Verification items for the finished model (mm, model axes). Face numbers are marked on the shaded views. Give positions to 0.01 mm unless a question says otherwise; leave off trailing zeros. Loops run counter-clockwise (first coordinate to the right, second up) from the corner with the lowest first, then second, coordinate; pieces in that order, holes last. Notation, with made-up numbers: M 14,14 L 63,14 A16 cw 63,43 Z; hole C 46.25,12.25 d8. An arc over 180 degrees is marked long. Put each result on its own line as item: value. Start each with the question number.
from build123d import *

# Parameters (mm, degrees)
F1_DEPTH = 10
F0_R     = 24.5
F2_DEPTH = 150
F4_D     = 8.5
F4_DEPTH = 31.001
F5_D     = 8.5
F6_DEPTH = 20
F7_DEPTH = 20


with BuildPart() as f1:
    # F0 (on Top) → F1 (new body)
    with BuildSketch(Plane.XY):
        with BuildLine():
            ThreePointArc((-9.06851449, 27.018735073), (0, 28.5), (9.06851449, 27.018735073))
            Line((9.06851449, 27.018735073), (9.8690700263, 29.3870967742))
            ThreePointArc((9.8690700263, 29.3870967742), (0, 31), (-9.8690700263, 29.3870967742))
            Line((-9.8690700263, 29.3870967742), (-9.06851449, 27.018735073))
        make_face()
        with BuildLine():
            ThreePointArc((-9.06851449, -27.018735073), (-28.5, 0), (-9.06851449, 27.018735073))
            Line((-9.06851449, 27.018735073), (-9.8690700263, 29.3870967742))
            ThreePointArc((-9.8690700263, 29.3870967742), (-31, 0), (-9.8690700263, -29.3870967742))
            Line((-9.8690700263, -29.3870967742), (-9.06851449, -27.018735073))
        make_face()
        with BuildLine():
            Line((9.8690700263, -29.3870967742), (9.06851449, -27.018735073))
            ThreePointArc((9.06851449, -27.018735073), (0, -28.5), (-9.06851449, -27.018735073))
            Line((-9.06851449, -27.018735073), (-9.8690700263, -29.3870967742))
            ThreePointArc((-9.8690700263, -29.3870967742), (0, -31), (9.8690700263, -29.3870967742))
        make_face()
        with BuildLine():
            ThreePointArc((9.06851449, 27.018735073), (23.1376604583, 16.6402724893), (28.5, 0))
            ThreePointArc((28.5, 0), (23.1376604583, -16.6402724893), (9.06851449, -27.018735073))
            Line((9.06851449, -27.018735073), (9.8690700263, -29.3870967742))
            ThreePointArc((9.8690700263, -29.3870967742), (25.1688415587, -18.0977737469), (31, 0))
            ThreePointArc((31, 0), (25.1688415587, 18.0977737469), (9.8690700263, 29.3870967742))
            Line((9.8690700263, 29.3870967742), (9.06851449, 27.018735073))
        make_face()
    extrude(amount=F1_DEPTH)

    # F0 (on Top) → F2 (join)
    with BuildSketch(Plane.XY):
        with BuildLine():
            ThreePointArc((9.06851449, -27.018735073), (23.1376604583, -16.6402724893), (28.5, 0))
            ThreePointArc((28.5, 0), (23.1376604583, 16.6402724893), (9.06851449, 27.018735073))
            ThreePointArc((9.06851449, 27.018735073), (0, 28.5), (-9.06851449, 27.018735073))
            ThreePointArc((-9.06851449, 27.018735073), (-28.5, 0), (-9.06851449, -27.018735073))
            ThreePointArc((-9.06851449, -27.018735073), (0, -28.5), (9.06851449, -27.018735073))
        make_face()
        Circle(F0_R, mode=Mode.SUBTRACT)
    extrude(amount=F2_DEPTH)

    # F4 (through all, one way)
    with BuildSketch(Plane.YZ):
        with Locations((0, 37.0021536946)):
            Circle(F4_D / 2)
    extrude(amount=-F4_DEPTH, mode=Mode.SUBTRACT)

    # F5 (through all)
    with Locations(Plane(origin=(0, 0, 0), x_dir=(0, 1, 0), z_dir=(-1, 0, 0))):
        with Locations((0, -37.0021536946)):
            Hole(F5_D / 2)

    # F0 (on Top) → F6 (join)
    with BuildSketch(Plane.XY):
        with BuildLine():
            ThreePointArc((-9.06851449, 27.018735073), (0, 28.5), (9.06851449, 27.018735073))
            Line((9.06851449, 27.018735073), (9.8690700263, 29.3870967742))
            ThreePointArc((9.8690700263, 29.3870967742), (0, 31), (-9.8690700263, 29.3870967742))
            Line((-9.8690700263, 29.3870967742), (-9.06851449, 27.018735073))
        make_face()
    extrude(amount=F6_DEPTH)

    # F0 (on Top) → F7 (join)
    with BuildSketch(Plane.XY):
        with BuildLine():
            Line((9.8690700263, -29.3870967742), (9.06851449, -27.018735073))
            ThreePointArc((9.06851449, -27.018735073), (0, -28.5), (-9.06851449, -27.018735073))
            Line((-9.06851449, -27.018735073), (-9.8690700263, -29.3870967742))
            ThreePointArc((-9.8690700263, -29.3870967742), (0, -31), (9.8690700263, -29.3870967742))
        make_face()
    extrude(amount=F7_DEPTH)


solid = f1.part
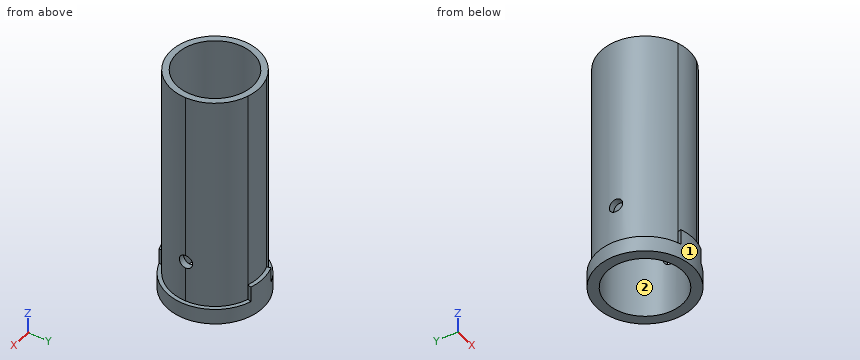
Q1. Cross-section at A-A, the plane x = 0. Record the boundary of the cut face in (y, z).
Q2. Cross-section at C-C, the plane z = 96. Record the boundary of the cut face in (x, y).
Q3. Release check for a two-part mould opening along Y. For the marked faces 1 and 2 record: pulls with the +Y half, pulls with the -Y half, needs draft (parallel to the pull), parting line crosses it, or undercut.
Q4. Cross-section at B-B, the plane y = -22.5. Record the boundary of the cut face in (x, z), then the cut area to 3 significant figures.
Q5. Cross-section at D-D, the plane x = -26.5. Record the boundary of the cut face in (y, z).
Q6. Go/stop test with flat-tipped pins: pin 1 (10 mm diameter, centred on x = -5, z = 41.5, fed in from +Y); pin 2 (24 mm diameter, centred on x = -15, y = 12.5, fed in from +Z); pin 3 (4 mm diameter, centred on y = 9.5, z = 56, fed in from +X); pin 4 (2 mm diameter, centred on x = 0, y = -30, fed in from +Z). Record where each tip stops, or that it passes through.
Q7. Scan lines: L1, parallel to Z at x = 26, y = 0; L2, parallel to Y at x = 0, z = 111; L3, parallel to Y at x = -14.5, z = 67. Record each from-to range of solid material in increasing order.
Ans:
1. outline: M -31,0 L -24.5,0 L -24.5,150 L -28.5,150 L -28.5,20 L -31,20 Z; M 24.5,0 L 31,0 L 31,20 L 28.5,20 L 28.5,150 L 24.5,150 Z
2. outline: C 0,0 d57; hole C 0,0 d49
3. face 1: parting line crosses it
3. face 2: undercut
4. outline: M -21.32,0 L -9.7,0 L -9.7,150 L -17.49,150 L -17.49,10 L -21.32,10 Z; M 9.7,0 L 21.32,0 L 21.32,10 L 17.49,10 L 17.49,150 L 9.7,150 Z
4. area: 2,420 mm^2
5. outline: M -16.09,0 L 16.09,0 L 16.09,10 L 10.49,10 L 10.49,150 L -10.49,150 L -10.49,10 L -16.09,10 Z; hole C 0,37 d8.5
6. pin 1: stops at y = 28.5
6. pin 2: stops at z = 150
6. pin 3: stops at x = 27.5
6. pin 4: stops at z = 20
7. L1: z = 0 to 32.75, 41.25 to 150
7. L2: y = -28.5 to -24.5, 24.5 to 28.5
7. L3: y = -24.54 to -19.75, 19.75 to 24.54
